Here's the drawing with two shaded views (mm, measured from the low corner). I have some questions. A direction names the side the tool comes from. Round coordinates to 2 decimals unless told otherwise and drop trailing zeros. Loops run counter-clockwise (first coordinate to the right, second up) from the corner with the lowest first, then second, coordinate; pieces in that order, holes last.
(1) Which directions (+Z, -Z, +X, -X, +Y, -Y) give clear straight access to the entire face, cutting with the end or side of a thin tool? Please do the marked faces 5 and 6.
(2) Will these pins go through, and if not, where does the flat tip stop? pin 1 Ø5 at (x, y) = (19, 15) entering from -Z; pin 2 Ø1.5 at (x, z) = (6, 19.5) entering from -Y; pin 3 Ø1 at (y, z) = (4.5, 20.5) entering from +X; pin 4 Ø3 at (x, z) = (9.5, 19) entering from +Y.
(3) Thinking about a two-plate mould opening in X: for the marked faces 1, 2, 3 and 4, which applies, released by +X, released by -X, zero draft, split by the parting line, or undercut?
(4) If I drill on line 1 along Y through (x, z) = (12.5, 16.5) (1 decimal); line 2 along X through (y, z) = (13.5, 23.25) (1 decimal); line 3 along Z through (x, y) = (6.75, 7), over which ranges is the centre line in solid material (lowest first)?
(5) I want a section at A-A on x = 15.75. Write out the boundary of the cut face in (y, z).
(6) I want a section at C-C on z = 18.75. Write out the boundary of the cut face in (x, y) (1 decimal).
(7) I want a section at B-B on y = 17.25. Write out the boundary of the cut face in (x, z), plus the area to 3 significant figures.
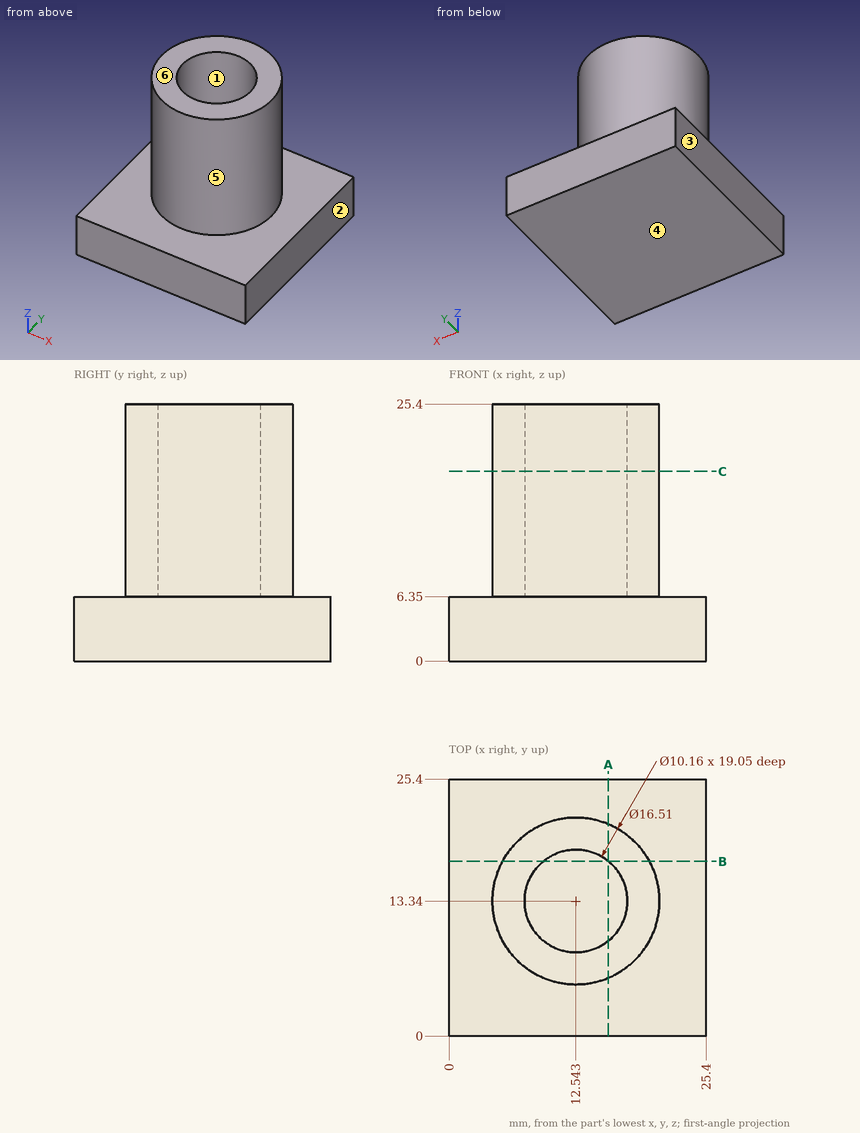
Filled sheet:
1. face 5: +Z
1. face 6: +Z, +X, -X, +Y, -Y
2. pin 1: stops at z = 0
2. pin 2: stops at y = 7.46
2. pin 3: passes through
2. pin 4: stops at y = 21.45
3. face 1: undercut
3. face 2: released by +X
3. face 3: released by -X
3. face 4: zero draft
4. line 1: y = 5.1 to 8.3, 18.4 to 21.6
4. line 2: x = 4.3 to 7.5, 17.6 to 20.8
4. line 3: z = 0 to 6.35
5. outline: (0, 0) - (25.4, 0) - (25.4, 6.35) - (20.95, 6.35) - (20.95, 25.4) - (17.28, 25.4) - (17.28, 6.35) - (9.4, 6.35) - (9.4, 25.4) - (5.73, 25.4) - (5.73, 6.35) - (0, 6.35) - close
6. outline: circle Ø16.5 at (12.5, 13.3); hole circle Ø10.2 at (12.5, 13.3)
7. outline: (0, 0) - (25.4, 0) - (25.4, 6.35) - (19.81, 6.35) - (19.81, 25.4) - (15.79, 25.4) - (15.79, 6.35) - (9.3, 6.35) - (9.3, 25.4) - (5.27, 25.4) - (5.27, 6.35) - (0, 6.35) - close
7. area: 315 mm2
